Drawing for the job (mm, zero at the part's lowest x, y, z). Give positions to 0.01 mm unless a question says otherwise; leave off trailing zeros. Order: outer loops, then holes, each group sorted by start corner. A loop starts at its lowest first (then second) coordinate and runs counter-clockwise, first axis right, second up. Notation, with made-up numbers: (78.25, 27.25) - (127.25, 27.25) arc R9 ccw to (127.25, 35.25) - close; hole circle Ø2 at (86.5, 44). An arc over 180 degrees is marked (long way). Use a Markdown table: item, result.
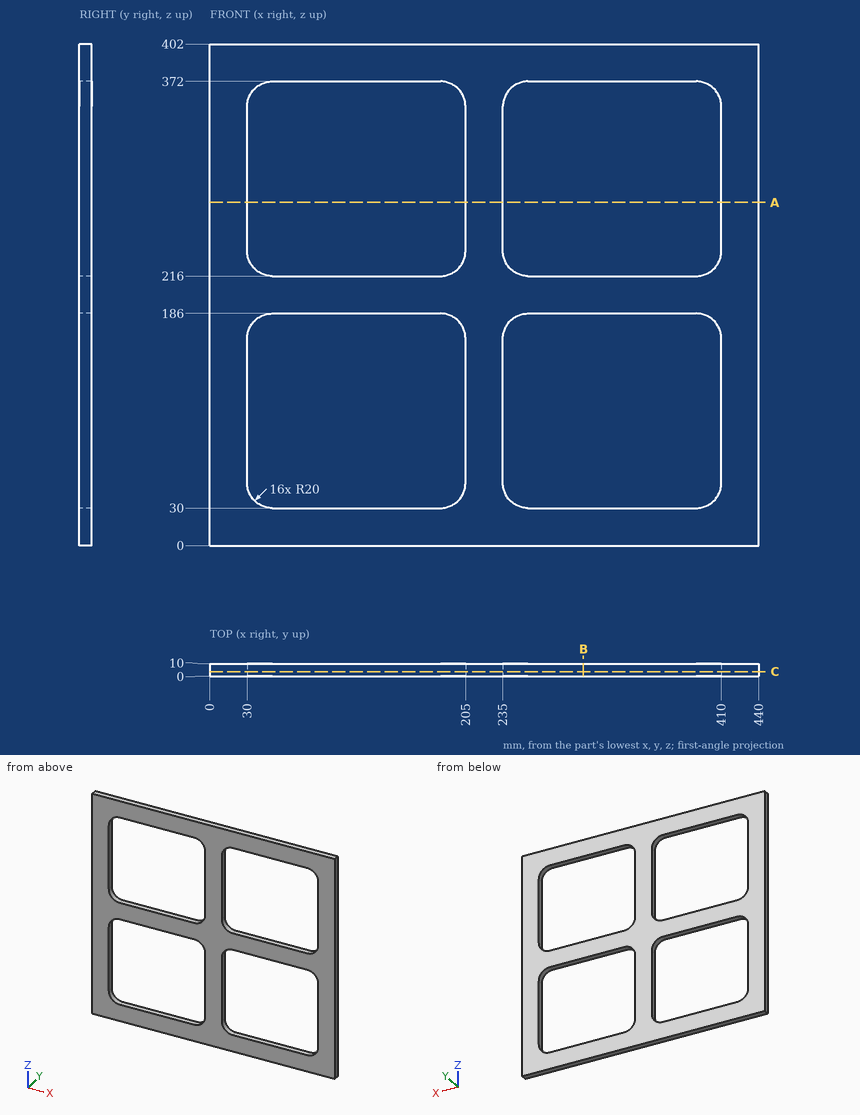
1) Slice it at A-A (z = 275). Write the cut outline in (x, y), and give its area (3 significant figures).
Computed:
| item | result |
|---|---|
| outline | (0, 0) - (30, 0) - (30, 10) - (0, 10) - close; (205, 0) - (235, 0) - (235, 10) - (205, 10) - close; (410, 0) - (440, 0) - (440, 10) - (410, 10) - close |
| area | 900 mm² |
2) Slice it at C-C (y = 3.5). State how many separate pieces and enclosed holes the cut face has, and give its area (3 significant figures).
Computed:
| item | result |
|---|---|
| separate pieces | 1 |
| enclosed holes | 4 |
| area | 69,100 mm² |
3) Pin check, flat tip, straight feed: P1, Ø3, axis at y = 7.5, z = 267.5, coming from the -X side. Stop position of the tip, or through.
Computed:
| item | result |
|---|---|
| P1 | stops at x = 0 |
4) Wall check: line 1 (X direction, y = 6.5, z = 165.5); line 2 (Z direction, x = 115, y = 6.5); line 3 (Z direction, x = 199, y = 5). Give the ranges that are in metal, low to high. Write a range as from..to.
Computed:
| item | result |
|---|---|
| line 1 | x = 0..30, 205..235, 410..440 |
| line 2 | z = 0..30, 186..216, 372..402 |
| line 3 | z = 0..35.72, 180.28..221.72, 366.28..402 |
5) Slice it at B-B (x = 299.5). Write the cut outline in (y, z).
Computed:
| item | result |
|---|---|
| outline | (0, 0) - (10, 0) - (10, 30) - (0, 30) - close; (0, 186) - (10, 186) - (10, 216) - (0, 216) - close; (0, 372) - (10, 372) - (10, 402) - (0, 402) - close |
